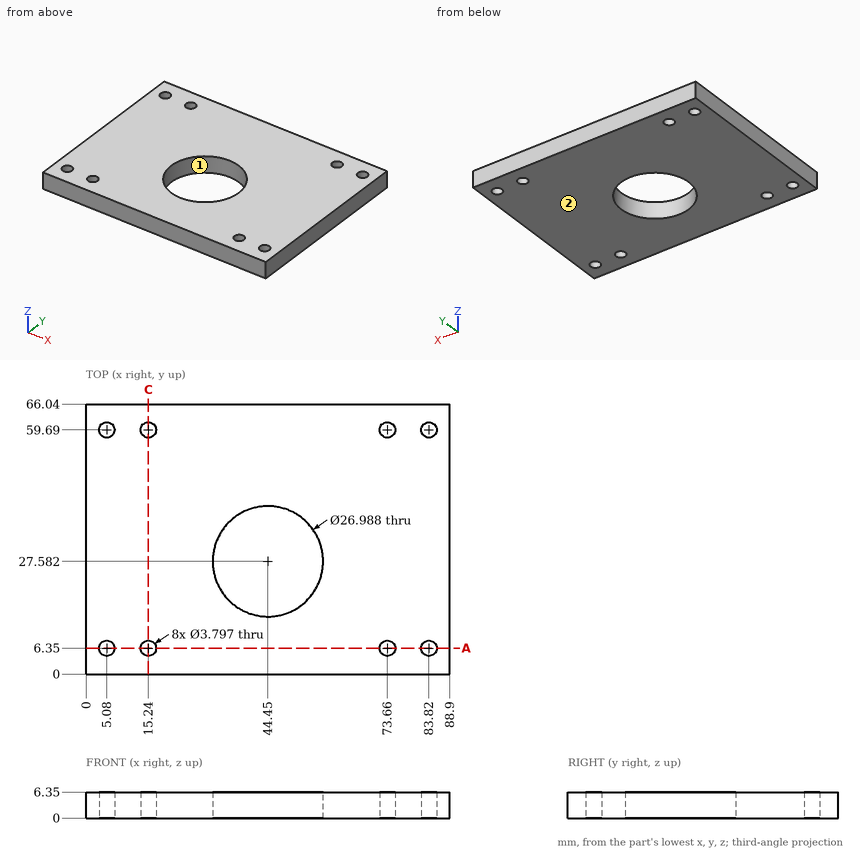
Verification items for this drawing (mm, ordinates from the low corner). Give positions to 0.01 mm unless a question says otherwise; leave off trailing zeros. Loops run counter-clockwise (first coordinate to the right, second up) from the corner with the lowest first, then second, coordinate; pieces in that order, holes last. Notation, with made-up numbers: (-40, -29) - (-9, -29) arc R33 cw to (-9, 1) - close; hole circle Ø3 at (83, 22). An arc over 180 degrees is marked (long way). Write item = value, one per line. Start each with the question number.
Q1. Cross-section at C-C, the plane x = 15.24. Enter the section's corners in (y, z).
Q2. Thickness scan on line 1 (Y direction, x = 15.24, z = 4.5); line 2 (X direction, y = 7, z = 3) (1 decimal); line 3 (Y direction, x = 37, z = 5). Record the ranges inside material, lowest first.
Q3. Cross-section at A-A, the plane y = 6.35. Enter the section's corners in (x, z), and give its area (3 significant figures).
Q4. Mould release check, pull along X, two halves, no side actions. Record for the marked faces 1 and 2: released by +X, released by -X, zero draft, split by the parting line, or undercut.
Q5. Depth check by flat-ended pin: P1, Ø2.5, axis at x = 5.08, y = 6.35, coming from the +Z side. Enter the tip coordinate at first touch or a pass-through.
Answer key:
q1.outline = (0, 0) - (4.45, 0) - (4.45, 6.35) - (0, 6.35) - close; (8.25, 0) - (57.79, 0) - (57.79, 6.35) - (8.25, 6.35) - close; (61.59, 0) - (66.04, 0) - (66.04, 6.35) - (61.59, 6.35) - close
q2.line_1 = 0 to 4.45, 8.25 to 57.79, 61.59 to 66.04
q2.line_2 = 0 to 3.3, 6.9 to 13.5, 17 to 71.9, 75.4 to 82, 85.6 to 88.9
q2.line_3 = 0 to 16.33, 38.83 to 66.04
q3.outline = (0, 0) - (3.18, 0) - (3.18, 6.35) - (0, 6.35) - close; (6.98, 0) - (13.34, 0) - (13.34, 6.35) - (6.98, 6.35) - close; (17.14, 0) - (71.76, 0) - (71.76, 6.35) - (17.14, 6.35) - close; (75.56, 0) - (81.92, 0) - (81.92, 6.35) - (75.56, 6.35) - close; (85.72, 0) - (88.9, 0) - (88.9, 6.35) - (85.72, 6.35) - close
q3.area = 468 mm^2
q4.face_1 = undercut
q4.face_2 = zero draft
q5.P1 = through
